Autodesk Inventor part; units mm, degrees
ref_plane "YZ Plane" through (0, 0, 0) normal (1, 0, 0) x (0, 1, 0)
ref_plane "XZ Plane" through (0, 0, 0) normal (0, 1, 0) x (-1, 0, 0)
ref_plane "XY Plane" through (0, 0, 0) normal (0, 0, 1) x (1, 0, 0)
sketch "Sketch1" plane through (0, 0, 0) normal (0, 1, 0) x (-1, 0, 0)
  circle A0 centre (0, 0) radius 40
  circle A1 centre (0, 0) radius 35
  line L0 (-0.75, -40) -> (-0.75, -35)
  line L1 (-23, -26.381812) -> (-23, -32.726136)
  line L2 (-34.93812, 2.828496) -> (-39.945867, 2.828496)
  line L3 (-39.945867, 1.33215) -> (-34.93812, 1.33215)
  line L4 (-24.132224, 25.315702) -> (-27.666452, 28.85856)
  line L5 (-26.660208, 29.866295) -> (-27.720868, 28.808219)
  line L6 (-39.940266, 2.933386) -> (-39.940266, 1.43704)
  line L7 (-23, -32.726136) -> (-21.5, -32.726136)
  circle A2 centre (0, 0) radius 42
  line L8 (-2.35, 40) -> (-2.35, 32.985933)
  line L9 (-27.666452, 28.85856) -> (-27.668423, 28.860536)
  line L10 (-26.660208, 29.866295) -> (-18.248408, 29.866295)
  line L11 (-21.5, -32.726136) -> (-12.409674, -32.726136)
  line L12 (-0.75, -35) -> (-0.75, -34.991963)
  line L13 (-34.93812, 2.828496) -> (-34.885522, 2.828496)
  line L14 (-39.945867, 1.33215) -> (-39.977811, 1.33215)
  line L15 (-39.940266, 1.43704) -> (-39.940266, 1.33215)
  line L16 (-0.75, -40) -> (-0.75, -41.993303)
  line L17 (-2.35, 40) -> (-2.35, 41.934204)
  line L18 (-39.892655, 2.928496) -> (-34.877269, 2.928496)
  line L19 (-34.978305, 1.23215) -> (-39.981018, 1.23215)
  line L20 (-39.892655, 2.928496) -> (-39.940266, 2.933386)
  point P0 (-24.149901, 25.333422)
  point P1 (-2.35, 34.921018)
  point P2 (-2.35, 39.930909)
  point P3 (-0.75, -39.992968)
  point P4 (-34.974639, 1.33215)
  point P5 (-39.89987, 2.828496)
  dimension "d0" = 2
  dimension "d3" = 0.1
  dimension "d4" = 0.1
sketch "Sketch1 outline for Extrusion1" plane through (0, 0, 0) normal (0, 1, 0) x (-1, 0, 0)
  line L0 (-27.666452, 28.85856) -> (-26.660208, 29.866295)
  line L1 (-24.149901, 25.333422) -> (-27.666452, 28.85856)
  arc A0 (-34.877269, 2.928496) -> (-24.149901, 25.333422) centre (0, 0) cw
  line L2 (-39.892655, 2.928496) -> (-34.877269, 2.928496)
  arc A1 (-39.981018, 1.23215) -> (-39.892655, 2.928496) centre (0, 0) cw
  line L3 (-34.978305, 1.23215) -> (-39.981018, 1.23215)
  arc A2 (-23, -26.381812) -> (-34.978305, 1.23215) centre (0, 0) cw
  line L4 (-23, -32.726136) -> (-23, -26.381812)
  line L5 (-21.5, -32.726136) -> (-23, -32.726136)
  line L6 (-12.409674, -32.726136) -> (-21.5, -32.726136)
  arc A3 (-0.75, -34.991963) -> (-12.409674, -32.726136) centre (0, 0) cw
  line L7 (-0.75, -35) -> (-0.75, -34.991963)
  line L8 (-0.75, -40) -> (-0.75, -35)
  line L9 (-0.75, -41.993303) -> (-0.75, -40)
  arc A4 (-2.35, 41.934204) -> (-0.75, -41.993303) centre (0, 0) ccw
  line L10 (-2.35, 40) -> (-2.35, 41.934204)
  line L11 (-2.35, 34.921018) -> (-2.35, 40)
  arc A5 (-18.248408, 29.866295) -> (-2.35, 34.921018) centre (0, 0) cw
  line L12 (-26.660208, 29.866295) -> (-18.248408, 29.866295)
extrude "Extrusion1" add sketch "Sketch1 outline for Extrusion1" along normal blind 3
equation "\"d4\" = slack"
equation "\"slack\" = 0.1"
properties part number "Back_front_aligner"
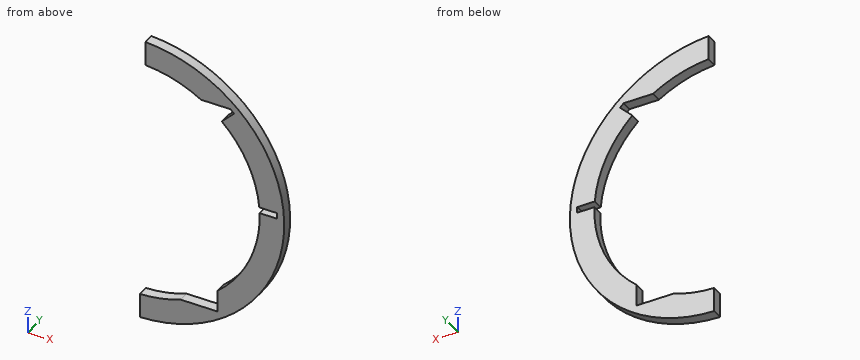
For this review, take the finished solid that the model builds, in its own axes (mm). Round coordinates to 2 decimals unless told otherwise and drop trailing zeros. Write each loop counter-clockwise with the first axis right and the second up, starting at its lowest first coordinate (ties: lowest second). Pieces come first, ordered by that corner, then holes. Notation, with made-up numbers: (21, 54) -> (50, 54) arc R16 ccw to (50, 72) -> close; hole circle Ø1 at (-8, -6.75). An arc over 180 degrees is marked (long way). Use one line per item in the form item = value.
1) Clearance check with flat-ended pins moving along their axes: pin 1 (1.5 mm diameter, centred on x = 38.5, y = 2, fed in from -Z); pin 2 (0.9 mm diameter, centred on x = 38.5, y = 1, fed in from +Z); pin 3 (1.5 mm diameter, centred on y = 1.5, z = -28, fed in from -X). State where each tip first meets the part, or that it passes through.
Found:
pin_1 = -18.41
pin_2 = 17.78
pin_3 = 23
2) To check wall thickness, follow L1, parallel to Z at x = 5, y = 0.8; L2, parallel to X at y = 0.25, z = 0; L3, parallel to Z at x = 7.5, y = 0.5. State the ranges of each line that lie inside material, in increasing order. Write a range as from..to.
Found:
L1 = -41.7..-34.64, 34.64..41.7
L2 = 35..42
L3 = -41.32..-34.19, 34.19..41.32
3) Take a section at B-B, the plane x = 6. Write out the cut boundary in (y, z).
Found:
outline = (0, -41.57) -> (3, -41.57) -> (3, -34.48) -> (0, -34.48) -> close; (0, 34.48) -> (3, 34.48) -> (3, 41.57) -> (0, 41.57) -> close
4) Take a section at C-C, the plane z = 0. Write out the cut boundary in (x, y), and give its area (3 significant figures).
Found:
outline = (35, 0) -> (42, 0) -> (42, 3) -> (35, 3) -> close
area = 21.0 mm2
5) Take a section at D-D, the plane x = 21.5. Write out the cut boundary in (y, z).
Found:
outline = (0, -36.08) -> (3, -36.08) -> (3, -32.73) -> (0, -32.73) -> close; (0, 29.87) -> (3, 29.87) -> (3, 36.08) -> (0, 36.08) -> close
